Can you work these out from the model? Positions are in its coordinate system, mm. A direction names the side the tool comes from. Give positions to 0.01 mm unless a question says otherwise; leave off trailing zeros. Loops run counter-clockwise (first coordinate to the right, second up) from the corner with the lowest first, then second, coordinate; pieces in that order, holes last.
from build123d import *

# Parameters (mm, degrees)
SKETCH1_W               = 89.4
SKETCH1_H               = 89.4
SKETCH1_R               = 0.95
BOSS_EXTRUDE1_DEPTH     = 2.5
SKETCH5_W               = 65
SKETCH5_H               = 74
BOSS_EXTRUDE3_DEPTH     = 2.5
SKETCH7_R               = 0.95
CUT_EXTRUDE2_DEPTH      = 4
CUT_EXTRUDE1_DEPTH      = 64.412774738
CUT_EXTRUDE1_DEPTH_BACK = 64.412774738
SKETCH2_W               = 12.2
SKETCH2_H               = 23
SKETCH2_W_2             = 52.6
SKETCH2_H_2             = 8.025
SKETCH2_W_3             = 23.1
SKETCH2_H_3             = 45.67
SKETCH2_H_4             = 43.68
SKETCH2_H_5             = 8.8
CHAMFER2_SIZE           = 1.3
CHAMFER3_SIZE           = 1.3
CHAMFER4_SIZE           = 1.7
CHAMFER5_SIZE           = 2.5


with BuildPart() as part:
    # Sketch1 → Boss-Extrude1 (new body)
    with BuildSketch(Plane(origin=(0, 0, 0), x_dir=(1, 0, 0), z_dir=(0, 1, 0))):
        Rectangle(SKETCH1_W, SKETCH1_H)
        with Locations(Location((-38.6, 38.3, 0), (0, 0, 270))):
            Circle(SKETCH1_R, mode=Mode.SUBTRACT)
        with Locations(Location((-38.6, 10.5, 0), (0, 0, 270))):
            Circle(SKETCH1_R, mode=Mode.SUBTRACT)
        with Locations(Location((-38.6, -10.5, 0), (0, 0, 270))):
            Circle(SKETCH1_R, mode=Mode.SUBTRACT)
        with Locations(Location((-38.6, -38.3, 0), (0, 0, 270))):
            Circle(SKETCH1_R, mode=Mode.SUBTRACT)
        with Locations(Location((38.6, -38.3, 0), (0, 0, 90))):
            Circle(SKETCH1_R, mode=Mode.SUBTRACT)
        with Locations(Location((38.6, -10.5, 0), (0, 0, 90))):
            Circle(SKETCH1_R, mode=Mode.SUBTRACT)
        with Locations(Location((38.6, 10.5, 0), (0, 0, 90))):
            Circle(SKETCH1_R, mode=Mode.SUBTRACT)
        with Locations(Location((38.6, 38.3, 0), (0, 0, 90))):
            Circle(SKETCH1_R, mode=Mode.SUBTRACT)
    extrude(amount=BOSS_EXTRUDE1_DEPTH)

    # Sketch5 → Boss-Extrude3 (add)
    with BuildSketch(Plane.XZ):
        Rectangle(SKETCH5_W, SKETCH5_H)
    extrude(amount=BOSS_EXTRUDE3_DEPTH)

    # Sketch7 → Cut-Extrude2 (cut)
    with BuildSketch(Plane(origin=(0, 2.5, 0), x_dir=(1, 0, 0), z_dir=(0, 1, 0))):
        with Locations(Location((-24.15, 18.595, 0), (0, 0, 270))):
            Circle(SKETCH7_R)
        with Locations(Location((24.15, 16.605, 0), (0, 0, 270))):
            Circle(SKETCH7_R)
        with Locations(Location((-19.07, -33.475, 0), (0, 0, 270))):
            Circle(SKETCH7_R)
        with Locations(Location((8.86, -33.475, 0), (0, 0, 270))):
            Circle(SKETCH7_R)
    extrude(amount=-CUT_EXTRUDE2_DEPTH, mode=Mode.SUBTRACT)

    # Sketch2 → Cut-Extrude1 (cut, two sides: drawn at the far end of the back side and taken through both)
    with BuildSketch(Plane(origin=(0, 2.5, 0), x_dir=(1, 0, 0), z_dir=(0, 1, 0)).offset(-CUT_EXTRUDE1_DEPTH_BACK)):
        with Locations((-38.6, 24.55)):
            Rectangle(SKETCH2_W, SKETCH2_H)
        Polygon((-26.3, 44.7), (26.3, 44.7), (26.3, 24.23), (26.3, 19.805), (0, 19.805), (0, 21.795), (-26.3, 21.795), align=None)
        with Locations((0, -40.6875)):
            Rectangle(SKETCH2_W_2, SKETCH2_H_2)
        with Locations((-14.75, -7.44)):
            Rectangle(SKETCH2_W_3, SKETCH2_H_3)
        with Locations((14.75, -8.435)):
            Rectangle(SKETCH2_W_3, SKETCH2_H_4)
        with Locations((-38.6, 0)):
            Rectangle(SKETCH2_W, SKETCH2_H_5)
        with Locations((38.6, 0)):
            Rectangle(SKETCH2_W, SKETCH2_H_5)
        with Locations((38.6, 24.55)):
            Rectangle(SKETCH2_W, SKETCH2_H)
        with Locations((38.6, -24.55)):
            Rectangle(SKETCH2_W, SKETCH2_H)
        with Locations((-38.6, -24.55)):
            Rectangle(SKETCH2_W, SKETCH2_H)
    extrude(amount=CUT_EXTRUDE1_DEPTH + CUT_EXTRUDE1_DEPTH_BACK, mode=Mode.SUBTRACT)

    # Chamfer2
    chamfer2_edges = [part.edges().sort_by_distance(p)[0] for p in [
        (0, 0, -21.795),
    ]]
    chamfer(chamfer2_edges, length=CHAMFER2_SIZE)

    # Chamfer3
    chamfer3_edges = [part.edges().sort_by_distance(p)[0] for p in [
        (-26.3, 0, -21.795),
        (26.3, 0, 36.675),
        (-26.3, 0, 36.675),
        (-26.3, 0, 30.275),
        (-3.2, 0, 30.275),
        (3.2, 0, 30.275),
        (26.3, 0, 30.275),
        (-3.2, 0, -15.395),
        (3.2, 0, -13.405),
        (26.3, 0, -13.405),
        (26.3, 0, -19.805),
        (-26.3, 0, -15.395),
    ]]
    chamfer(chamfer3_edges, length=CHAMFER3_SIZE)

    # Chamfer4
    chamfer4_edges = [part.edges().sort_by_distance(p)[0] for p in [
        (26.3, 1.25, 44.7),
        (-26.3, 1.25, 44.7),
        (-44.7, 1.25, 4.4),
        (-44.7, 1.25, -4.4),
        (-26.3, 1.25, -44.7),
        (26.3, 1.25, -44.7),
        (44.7, 1.25, -4.4),
        (44.7, 1.25, 4.4),
        (-44.7, 1.25, -44.7),
        (44.7, 1.25, -44.7),
        (44.7, 1.25, 44.7),
        (-44.7, 1.25, 44.7),
    ]]
    chamfer(chamfer4_edges, length=CHAMFER4_SIZE)

    # Chamfer5
    chamfer5_edges = [part.edges().sort_by_distance(p)[0] for p in [
        (28.9125, -2.5, 37),
        (29.4, -2.5, -37),
        (-29.4, -2.5, -37),
    ]]
    chamfer(chamfer5_edges, length=CHAMFER5_SIZE - 0.0001)  # a hair under: the kernel refuses the full size


solid = part.part
(1) Please list where these lines run through material, in increasing order: probe 1 along X at (y, z) = (2, 12); probe 2 along X at (y, z) = (0.55, -10.5); probe 3 along X at (y, z) = (2.25, 21.5).
Returned:
probe 1: x = -44.7 to -26.3, -3.2 to 3.2, 26.3 to 44.7
probe 2: x = -44.7 to -39.55, -37.65 to -26.3, -3.2 to 3.2, 26.3 to 37.65, 39.55 to 44.7
probe 3: x = -32.5 to -26.3, -3.2 to 3.2, 26.3 to 32.5
(2) Which directions (+Z, -Z, +X, -X, +Y, -Y) give clear straight access to the entire face, cutting with the end or side of a thin tool? Please do faces 4 (the flat face through (39, 1, 36.05)), 5 (the flat face through (0, 1, 36.675)), 6 (the flat face through (-26.3, 0, 8)), 7 (the flat face through (-19, -1.5, 33)), 8 (the flat face through (-39, 0, 9)).
Returned:
face 4: +X, +Y, -Y
face 5: +Z, +Y, -Y
face 6: +Y, -Y
face 7: +Y
face 8: +Z, -Z, -X, -Y
(3) Suppose I cut it at B-B on y = 1.6. Give the number of separate pieces and of enclosed holes in the cut face, plus the area to 3 significant figures.
Returned:
separate pieces: 1
enclosed holes: 14
area: 2,870 mm2
(4) Suppose I cut it at A-A on z = -2.5. List the corners of the cut face in (x, y) for me, plus the area to 3 significant figures.
Returned:
outline: (-32.5, -2.5) - (-26.3, -2.5) - (-26.3, 2.5) - (-32.5, 2.5) - close; (-3.2, -2.5) - (3.2, -2.5) - (3.2, 2.5) - (-3.2, 2.5) - close; (26.3, -2.5) - (32.5, -2.5) - (32.5, 2.5) - (26.3, 2.5) - close
area: 94.0 mm2
(5) Thinking about a two-plate mould opening in Z: for faces 1 (the flat face through (35, 1, 44.7)), 2 (the flat face through (-32.5, 0, -1)), 3 (the flat face through (26.3, 1, 41)), which applies, pulls with the +Z half, pulls with the -Z half, needs draft (parallel to the pull), parting line crosses it, or undercut?
Returned:
face 1: pulls with the +Z half
face 2: undercut
face 3: needs draft
(6) Will these pins go through, and if not, where does the flat tip stop? P1, Ø3, axis at y = 2, z = 24.5, coming from the -X side; P2, Ø2, axis at x = -38.6, z = 10.5, coming from the -Y side; P3, Ø9.5, axis at x = 34, z = -40.5, coming from the -Y side; P4, Ø6, axis at x = 13, z = -9.5, coming from the -Y side.
Returned:
P1: stops at x = -32.5
P2: stops at y = 0
P3: stops at y = -1.01
P4: passes through
